```python
from build123d import *

# Parameters (mm, degrees)
SKETCH1_W             = 10
SKETCH1_H             = 10
SKETCH1_R             = 1.5
BOSS_EXTRUDE1_DEPTH   = 2
BOSS_EXTRUDE1_2_DEPTH = 2
BOSS_EXTRUDE1_3_DEPTH = 2
BOSS_EXTRUDE1_4_DEPTH = 2
SKETCH2_W             = 68.718732211
SKETCH2_H             = 36.837925628
SKETCH2_R             = 1.5
BOSS_EXTRUDE2_DEPTH   = 2
SKETCH3_W             = 62.76
SKETCH3_H             = 45
SKETCH3_R             = 1.5
BOSS_EXTRUDE3_DEPTH   = 2
SKETCH4_R             = 1.5
CUT_EXTRUDE1_DEPTH    = 2
SKETCH5_R             = 1.5
CUT_EXTRUDE2_DEPTH    = 2
SKETCH6_R             = 1.538732211
CUT_EXTRUDE3_DEPTH    = 4
SKETCH7_W             = 53.44
SKETCH7_H             = 43.3
SKETCH7_R             = 1.5
BOSS_EXTRUDE4_DEPTH   = 2


with BuildPart() as part:
    # Sketch1 → Boss-Extrude1 (new body)
    with BuildSketch(Plane(origin=(0, 0, 0), x_dir=(1, 0, 0), z_dir=(0, 1, 0))):
        with Locations((-68.417052022, 33.167885028)):
            Rectangle(SKETCH1_W, SKETCH1_H)
        with Locations((-68.417052022, 33.167885028)):
            Circle(SKETCH1_R, mode=Mode.SUBTRACT)
    extrude(amount=BOSS_EXTRUDE1_DEPTH)



with BuildPart() as body_2:
    # Sketch1 → Boss-Extrude1 2 (new body)
    with BuildSketch(Plane(origin=(0, 0, 0), x_dir=(1, 0, 0), z_dir=(0, 1, 0))):
        with Locations((-68.356859369, 6.212274972)):
            Rectangle(SKETCH1_W, SKETCH1_H)
        with Locations((-68.356859369, 6.212274972)):
            Circle(SKETCH1_R, mode=Mode.SUBTRACT)
    extrude(amount=BOSS_EXTRUDE1_2_DEPTH)


with BuildPart() as body_3:
    # Sketch1 → Boss-Extrude1 3 (new body)
    with BuildSketch(Plane(origin=(0, 0, 0), x_dir=(1, 0, 0), z_dir=(0, 1, 0))):
        with Locations((-9.698319811, 6.3299594)):
            Rectangle(SKETCH1_W, SKETCH1_H)
        with Locations((-9.698319811, 6.3299594)):
            Circle(SKETCH1_R, mode=Mode.SUBTRACT)
    extrude(amount=BOSS_EXTRUDE1_3_DEPTH)


with BuildPart() as body_4:
    # Sketch1 → Boss-Extrude1 4 (new body)
    with BuildSketch(Plane(origin=(0, 0, 0), x_dir=(1, 0, 0), z_dir=(0, 1, 0))):
        with Locations((-9.698319811, 32.974349344)):
            Rectangle(SKETCH1_W, SKETCH1_H)
        with Locations((-9.698319811, 32.974349344)):
            Circle(SKETCH1_R, mode=Mode.SUBTRACT)
    extrude(amount=BOSS_EXTRUDE1_4_DEPTH)


with BuildPart() as part_1:
    add(part.part)

    add(body_2.part)  # Boss-Extrude2 merges body 2

    add(body_3.part)  # Boss-Extrude2 merges body 3

    add(body_4.part)  # Boss-Extrude2 merges body 4
    # Sketch2 → Boss-Extrude2 (add)
    with BuildSketch(Plane(origin=(0, 2, 0), x_dir=(1, 0, 0), z_dir=(0, 1, 0))):
        with Locations((-39.057685917, 19.748922214)):
            Rectangle(SKETCH2_W, SKETCH2_H)
        with Locations((-68.417052022, 33.167885028)):
            Circle(SKETCH2_R, mode=Mode.SUBTRACT)
        with Locations((-9.698319811, 32.974349344)):
            Circle(SKETCH2_R, mode=Mode.SUBTRACT)
        with Locations((-9.698319811, 6.3299594)):
            Circle(SKETCH2_R, mode=Mode.SUBTRACT)
        with Locations((-68.356859369, 6.212274972)):
            Circle(SKETCH2_R, mode=Mode.SUBTRACT)
    extrude(amount=BOSS_EXTRUDE2_DEPTH)

    # Sketch3 → Boss-Extrude3 (add)
    with BuildSketch(Plane(origin=(0, 4, 0), x_dir=(1, 0, 0), z_dir=(0, 1, 0))):
        with Locations((-40.297052022, 13.817885028)):
            Rectangle(SKETCH3_W, SKETCH3_H)
        with Locations((-68.417052022, 33.167885028)):
            Circle(SKETCH3_R, mode=Mode.SUBTRACT)
        with Locations((-68.356859369, 6.212274972)):
            Circle(SKETCH3_R, mode=Mode.SUBTRACT)
    extrude(amount=-BOSS_EXTRUDE3_DEPTH)

    # Sketch4 → Cut-Extrude1 (cut)
    with BuildSketch(Plane(origin=(0, 4, 0), x_dir=(1, 0, 0), z_dir=(0, 1, 0))):
        with Locations((-9.698319811, 6.3299594)):
            Circle(SKETCH4_R)
        with Locations((-9.698319811, 32.974349344)):
            Circle(SKETCH4_R)
    extrude(amount=-CUT_EXTRUDE1_DEPTH, mode=Mode.SUBTRACT)

    # Sketch5 → Cut-Extrude2 (cut)
    with BuildSketch(Plane(origin=(0, 4, 0), x_dir=(1, 0, 0), z_dir=(0, 1, 0))):
        with Locations((-68.417052022, -5.782114972)):
            Circle(SKETCH5_R)
        with Locations((-14.737052022, -5.782114972)):
            Circle(SKETCH5_R)
        with Locations((-14.737052022, 33.417885028)):
            Circle(SKETCH5_R)
    extrude(amount=-CUT_EXTRUDE2_DEPTH, mode=Mode.SUBTRACT)

    # Sketch6 → Cut-Extrude3 (cut)
    with BuildSketch(Plane(origin=(0, 4, 0), x_dir=(1, 0, 0), z_dir=(0, 1, 0))):
        with Locations((-14.698319811, 33.417885028)):
            Circle(SKETCH6_R)
    extrude(amount=-CUT_EXTRUDE3_DEPTH, mode=Mode.SUBTRACT)

    # Sketch7 → Boss-Extrude4 (add)
    with BuildSketch(Plane(origin=(0, 4, 0), x_dir=(1, 0, 0), z_dir=(0, 1, 0))):
        with Locations((-40.531724845, -40.332114972)):
            Rectangle(SKETCH7_W, SKETCH7_H)
        with Locations((-63.151724845, -22.532114972)):
            Circle(SKETCH7_R, mode=Mode.SUBTRACT)
        with Locations((-63.151724845, -58.132114972)):
            Circle(SKETCH7_R, mode=Mode.SUBTRACT)
        with Locations((-17.651724845, -58.232114972)):
            Circle(SKETCH7_R, mode=Mode.SUBTRACT)
        with Locations((-17.651724845, -22.432114972)):
            Circle(SKETCH7_R, mode=Mode.SUBTRACT)
        Polygon((-71.677052022, -18.682114972), (-67.251724845, -18.682114972), (-13.811724845, -18.682114972), (-8.917052022, -18.682114972), (-8.917052022, -8.682114972), (-71.677052022, -8.682114972), align=None)
    extrude(amount=-BOSS_EXTRUDE4_DEPTH)


solid = part_1.part
```
The listing builds one solid part. Answer for the finished solid, in the listing's coordinates (mm). A direction names the side the tool comes from. Give positions to 0.01 mm unless a question says otherwise; leave off trailing zeros. Order: outer loops, then holes, each group sorted by start corner. A loop starts at its lowest first (then second) coordinate and runs counter-clockwise, first axis right, second up. Notation, with made-up numbers: (81, 7) - (121, 7) arc R23 ccw to (121, 46) - close; hole circle Ø8 at (-5.5, -27). An arc over 180 degrees is marked (long way). Use one line per item in the form item = value. Start each with the question number.
(1) A cutting plane is placed at B-B, the plane z = 11. Write down the section's boundary in (x, y).
(2) For faces 1 (the flat face through (-10, 1, -27.974)), 2 (the flat face through (-68, 1, -1.212)), 3 (the flat face through (-10, 1, -37.974)), determine the directions among +Z, -Z, +X, -X, +Y, -Y from which every point of the face is accessible in a straight line to the end or side of a thin tool.
(3) A cutting plane is placed at C-C, the plane x = -53.5. Write down the section's boundary in (y, z), then the cut area to 3 significant figures.
(4) A cutting plane is placed at A-A, the plane y = 0.6. Write down the section's boundary in (x, z), then the cut area to 3 significant figures.
(5) Consider line 1 (Z direction, x = -67.5, y = 1.95); line 2 (Z direction, x = -67.5, y = 3.4); line 3 (Z direction, x = -65.5, y = 0.2). Determine where each line is inside the solid, lowest interval first. Write a range as from..to.
(6) Flat-ended cylindrical pins translate along their axes: pin 1 Ø2 at (y, z) = (3, 32.5) entering from +X; pin 2 Ø1 at (x, z) = (-41.5, 29.5) entering from -Y; pin 3 Ø2.5 at (x, z) = (-9.7, -32.97) entering from -Y; pin 4 Ø1 at (x, y) = (-68.5, 1) entering from +Z. Find the tip coordinate at first contact, or state that the pin passes through.
(7) The mould has two halves that part along X. Classify faces 4 (the cylindrical face through (-13.277, 2.472, -32.829)), 5 (the flat face through (-14.698, 1, -6)), 6 (the flat face through (-40, 3, -38.168)), 7 (the flat face through (-67.252, 3, 41)): released by +X, released by -X, zero draft, split by the parting line, or undercut.
Ans:
q1.outline = (-71.68, 2) - (-8.92, 2) - (-8.92, 4) - (-71.68, 4) - close
q2.face_1 = +X, -X, -Y
q2.face_2 = +Z, +X, -X, -Y
q2.face_3 = -Z, +X, -Y
q3.outline = (2, -38.17) - (4, -38.17) - (4, 61.98) - (2, 61.98) - close
q3.area = 200 mm^2
q4.outline = (-73.42, -38.17) - (-63.42, -38.17) - (-63.42, -28.17) - (-73.42, -28.17) - close; (-73.36, -11.21) - (-63.36, -11.21) - (-63.36, -1.21) - (-73.36, -1.21) - close; (-14.7, -37.97) - (-4.7, -37.97) - (-4.7, -27.97) - (-14.7, -27.97) - (-14.7, -31.88) arc R1.54 cw to (-14.7, -34.96) - close; (-14.7, -11.33) - (-4.7, -11.33) - (-4.7, -1.33) - (-14.7, -1.33) - close; hole circle Ø3 at (-68.42, -33.17); hole circle Ø3 at (-68.36, -6.21); hole circle Ø3 at (-9.7, -32.97); hole circle Ø3 at (-9.7, -6.33)
q4.area = 368 mm^2
q5.line_1 = -38.17..-34.35, -31.98..-28.17, -11.21..-7.44, -4.98..-1.21
q5.line_2 = -38.17..-34.35, -31.98..-7.44, -4.98..4.6, 6.97..18.68
q5.line_3 = -38.17..-28.17, -11.21..-1.21
q6.pin_1 = -13.81
q6.pin_2 = 2
q6.pin_3 = through
q6.pin_4 = -1.21
q7.face_4 = undercut
q7.face_5 = undercut
q7.face_6 = zero draft
q7.face_7 = released by -X
